Autodesk Inventor part; units mm, degrees
ref_plane "YZ Plane" through (0, 0, 0) normal (1, 0, 0) x (0, 1, 0)
ref_plane "XZ Plane" through (0, 0, 0) normal (0, 1, 0) x (-1, 0, 0)
ref_plane "XY Plane" through (0, 0, 0) normal (0, 0, 1) x (1, 0, 0)
sketch "Sketch1" plane through (0, 0, 0) normal (0, 0, 1) x (1, 0, 0)
  line L0 (0, 0) -> (12.7, 0)
  line L1 (12.7, 0) -> (12.7, -11.9296)
  line L2 (0, 0) -> (0, -12.7)
  line L3 (0, -12.7) -> (14.4801, -27.1801)
  arc A0 (14.4801, -27.1801) -> (21.2153, -20.4449) centre (17.8477, -23.8125) ccw
  line L4 (21.2153, -20.4449) -> (12.7, -11.9296)
  dimension "d10" = 12.7
  dimension "d11" = 12.7
  dimension "d12" = 45
  dimension "d13" = 23.8125
  dimension "d14" = 4.7625
extrude "Extrusion1" add sketch "Sketch1" along normal blind 3
sketch "Sketch2" plane through (0, 0, 3) normal (0, 0, 1) x (1, 0, 0)
  line L0 (12.7, 0) -> (12.7, -11.9296)
  line L1 (0, 0) -> (12.7, 0)
  line L2 (0, -12.7) -> (0, 0)
  line L3 (0, -3) -> (12.7, -3)
  dimension "d17" = 3
extrude "Extrusion2" add sketch "Sketch2" along normal blind 9.525
sketch "Sketch3" plane through (0, 0, 0) normal (0, 1, 0) x (1, 0, 0)
  line L0 (0, 0) -> (0, -12.525)
  line L1 (0, -12.525) -> (12.7, -12.525)
  point P0 (6.35, -7.7625)
  dimension "d20" = 4.7625
  dimension "d21" = 6.35
hole "Hole1" at (6.35, 0, 7.7625) direction (0, -1, 0) diameter 3.175 end through all
sketch "Sketch4" plane through (0, 0, 0) normal (0, 0, -1) x (-1, 0, 0)
  arc A0 (-21.2153, -20.4449) -> (-14.4801, -27.1801) centre (-17.8477, -23.8125) ccw
hole "Hole2" at (17.8477, -23.8125, 0) direction (0, 0, 1) diameter 4.826 end through all
properties part number "PWTR-0043" material "Stainless Steel, 303"
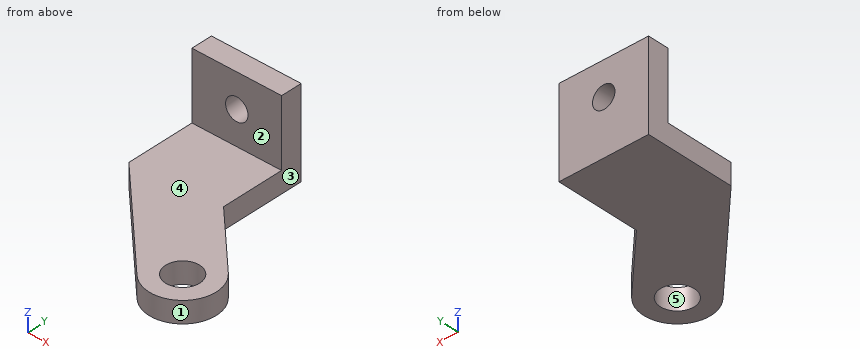
Build history of the part. All positions in model axes, mm. Face numbers are marked on the shaded views. A direction names the side the tool comes from. Round coordinates to 2 decimals unless told otherwise and drop trailing zeros. Order: outer loops, then holes, each group sorted by start corner. A loop starts at its lowest first (then second) coordinate and runs counter-clockwise, first axis right, second up. Notation, with made-up numbers: (67.5, 42.25) - (90.5, 42.25) arc R16 cw to (90.5, 57.25) - close; hole circle Ø2 at (-1.75, 74). An arc over 180 degrees is marked (long way). Use a Markdown table: item, result.
1) Saw through at B-B on z = 6.5. Write the cut outline in (x, y).
Recorded:
| item | result |
|---|---|
| outline | (0, -3) - (5.39, -3) - (5.39, 0) - (0, 0) - close; (7.31, -3) - (12.7, -3) - (12.7, 0) - (7.31, 0) - close |
2) Saw through at D-D on y = -9. Write the cut outline in (x, z), and give its area (3 significant figures).
Recorded:
| item | result |
|---|---|
| outline | (0, 0) - (12.7, 0) - (12.7, 3) - (0, 3) - close |
| area | 38.1 mm² |
3) Saw through at A-A on x = 6.35. Write the cut outline in (y, z) (3 decimals), and give its area (3 significant figures).
Recorded:
| item | result |
|---|---|
| outline | (-19.05, 0) - (0, 0) - (0, 6.175) - (-3, 6.175) - (-3, 3) - (-19.05, 3) - close; (-3, 9.35) - (0, 9.35) - (0, 12.525) - (-3, 12.525) - close |
| area | 76.2 mm² |
4) Wall check: L1, parallel to Y at x = 7.25, z = 12.25; L2, parallel to Z at x = 6.35, y = -1.9 (3 decimals); L3, parallel to X at y = -24.75, z = 1. Give the ranges that are in metal, low to high.
Recorded:
| item | result |
|---|---|
| L1 | y = -3 to 0 |
| L2 | z = 0 to 6.175, 9.35 to 12.525 |
| L3 | x = 12.05 to 15.62, 20.07 to 22.52 |
5) Flat gauge pins, fed straight in: pin 1 Ø6.5 at (x, y) = (17.85, -23.81) entering from -Z; pin 2 Ø6 at (x, z) = (14, 9.5) entering from -Y; pin 3 Ø11.5 at (x, y) = (7, -14.5) entering from +Z; pin 4 Ø1 at (y, z) = (-15.5, 2) entering from +X. Where does each tip first touch, or does it go through?
Recorded:
| item | result |
|---|---|
| pin 1 | stops at z = 0 |
| pin 2 | stops at y = -3 |
| pin 3 | stops at z = 3 |
| pin 4 | stops at x = 16.77 |
6) Saw through at C-C on x = 10.25. Write the cut outline in (y, z) (3 decimals).
Recorded:
| item | result |
|---|---|
| outline | (-22.95, 0) - (0, 0) - (0, 12.525) - (-3, 12.525) - (-3, 3) - (-22.95, 3) - close |
7) Pull direction X, two halves, no side cores. Call the marked faces 3, 4 and 5: pulls with the +X half, pulls with the -X half, needs draft (parallel to the pull), parting line crosses it, or undercut.
Recorded:
| item | result |
|---|---|
| face 3 | pulls with the +X half |
| face 4 | needs draft |
| face 5 | undercut |
8) Tool access for the marked faces 1 and 2: list every direction of +Z, -Z, +X, -X, +Y, -Y with a clear straight run to the whole face (end or side of a thin tool).
Recorded:
| item | result |
|---|---|
| face 1 | +Z, -Z |
| face 2 | +Z, +X, -X, -Y |
